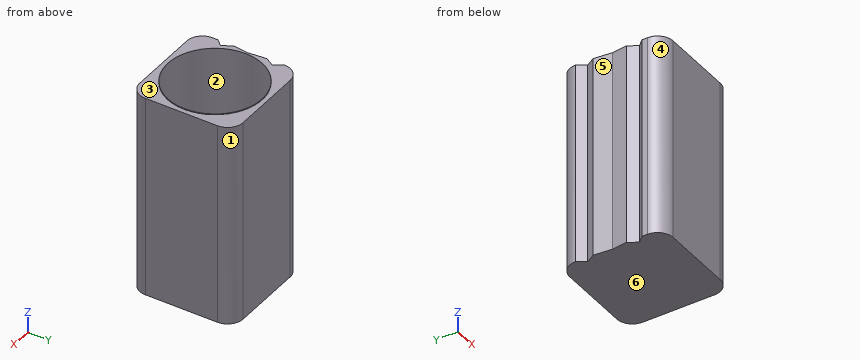
```python
from build123d import *

# Parameters (mm, degrees)
F0_W     = 0.1
F0_H     = 65
F2_R     = 15.1
F3_DEPTH = 64.8
F4_R     = 15.089878
F5_DEPTH = 4


with BuildPart() as f1:
    # F0 (on Front) → F1 (revolve)
    with BuildSketch(Plane.XZ):
        with Locations((-15.05, 32.5)):
            Rectangle(F0_W, F0_H)
    revolve(axis=Axis((0, 0, 13.169291), (0, 0, 1)))

    # F2 (on Top) → F3 (join)
    with BuildSketch(Plane.XY):
        with BuildLine():
            Line((-11.5, -16.5), (11.5, -16.5))
            ThreePointArc((11.5, -16.5), (15.035534, -15.035534), (16.5, -11.5))
            Line((16.5, -11.5), (16.5, 11.5))
            ThreePointArc((16.5, 11.5), (15.035534, 15.035534), (11.5, 16.5))
            Line((11.5, 16.5), (-11.509184, 16.5))
            ThreePointArc((-11.509184, 16.5), (-15.07744, 15.002506), (-16.508319, 11.407019))
            Line((-16.508319, 11.407019), (-14.724482, 8.708321))
            Line((-14.724482, 8.708321), (-16.424482, 5.869184))
            Line((-16.424482, 5.869184), (-15.872665, 0))
            Line((-15.872665, 0), (-16.470676, -4.755567))
            Line((-16.470676, -4.755567), (-14.637756, -7.762516))
            Line((-14.637756, -7.762516), (-16.492511, -9.777418))
            Line((-16.492511, -9.777418), (-16.5, -11.5))
            ThreePointArc((-16.5, -11.5), (-15.035534, -15.035534), (-11.5, -16.5))
        make_face()
        Circle(F2_R, mode=Mode.SUBTRACT)
    extrude(amount=F3_DEPTH)

    # F4 (on Top) → F5 (join)
    with BuildSketch(Plane.XY):
        Circle(F4_R)
    extrude(amount=F5_DEPTH)


solid = f1.part
```
The model under review builds one solid part; all positions refer to its coordinate system, in mm. Face numbers are marked on the shaded views. A direction names the side the tool comes from. Round coordinates to 2 decimals unless told otherwise and drop trailing zeros. Loops run counter-clockwise (first coordinate to the right, second up) from the corner with the lowest first, then second, coordinate; pieces in that order, holes last. Notation, with made-up numbers: M 86.5,-13 L 139.5,-13 A34 cw 139.5,22 Z; hole C 23,43.5 d1. An arc over 180 degrees is marked long. Put each result on its own line as item: value.
Q1. Mouldability with a two-part tool opening along X and no side actions: class the marked faces 1, 2, 3 and 4 as released by +X, released by -X, zero draft, split by the parting line, or undercut.
Result set:
face 1: released by +X
face 2: undercut
face 3: zero draft
face 4: released by -X
Q2. Consider section A-A, the plane z = 6. Give the boundary of the cut face in (x, y).
Result set:
outline: M -16.51,11.41 L -14.72,8.71 L -16.42,5.87 L -15.87,0 L -16.47,-4.76 L -14.64,-7.76 L -16.49,-9.78 L -16.5,-11.5 A5 ccw -11.5,-16.5 L 11.5,-16.5 A5 ccw 16.5,-11.5 L 16.5,11.5 A5 ccw 11.5,16.5 L -11.51,16.5 A5 ccw Z; hole C 0,0 d30
Q3. For pin 1 (4 mm diameter, centred on x = -0.5, y = 6.5, fed in from +Z); pin 2 (1.5 mm diameter, centred on y = -1, z = 57.5, fed in from -X); pin 3 (1 mm diameter, centred on y = -8, z = 25, fed in from -X), all flat-tipped, find the tip position at first contact; note any pin that passes through.
Result set:
pin 1: stops at z = 4
pin 2: stops at x = -16.09
pin 3: stops at x = -15.32
Q4. Consider section C-C, the plane y = 5. Give the boundary of the cut face in (x, z).
Result set:
outline: M -16.34,0 L 16.5,0 L 16.5,64.8 L 14.25,64.8 L 14.25,65 L 14.14,65 L 14.14,4 L -14.14,4 L -14.14,65 L -14.25,65 L -14.25,64.8 L -16.34,64.8 Z
Q5. To check wall thickness, follow L1, parallel to Y at x = 0, z = 47.5; L2, parallel to X at y = 0, z = 36; L3, parallel to Z at x = 6, y = 8. State the ranges of each line that lie inside material, in increasing order.
Result set:
L1: y = -16.5 to -15, 15 to 16.5
L2: x = -15.87 to -15, 15 to 16.5
L3: z = 0 to 4
Q6. Machinability: for the marked faces 5 and 6, which of the approach directions +Z, -Z, +X, -X, +Y, -Y give a long, thin tool a straight path to every point of the face, cutting with its end or side? Answer none if there is none.
Result set:
face 5: +Z, -Z, -X
face 6: -Z, +X, -X, +Y, -Y
Q7. Consider section B-B, the plane x = 0. Give the boundary of the cut face in (y, z).
Result set:
outline: M -16.5,0 L 16.5,0 L 16.5,64.8 L 15.1,64.8 L 15.1,65 L 15,65 L 15,4 L -15,4 L -15,65 L -15.1,65 L -15.1,64.8 L -16.5,64.8 Z
